Design review of the part built by this model. Coordinates are the model's own, in mm. Round coordinates to 2 decimals unless told otherwise and drop trailing zeros. Order: outer loops, then holes, each group sorted by start corner. A loop starts at its lowest first (then second) coordinate and runs counter-clockwise, first axis right, second up. Notation, with made-up numbers: M -24,57 L 22,57 A17 ccw 22,72 Z; hole C 69,-33 d10. An arc over 180 degrees is marked long. Use a Markdown table: item, result. Add a question column.
(1) Take a section at A-A (x = -104.5). Write out the cut boundary in (y, z).
(2) For pin 1 (3 mm diameter, centred on y = -21.5, z = 4, fed in from +X); pin 2 (3 mm diameter, centred on x = 296.5, z = 2, fed in from -Y), all flat-tipped, find the tip position at first contact; note any pin that passes through.
(3) To check wall thickness, follow probe 1 along X at (y, z) = (11, 3.75); probe 2 along Y at (x, z) = (196, 1.8); probe 3 along X at (y, z) = (-14.5, 4.55). State the ranges of each line that lie inside material, in increasing order. Write a range as from..to.
(4) Take a section at B-B (z = 3). Count the separate pieces of the cut face and the enclosed holes in it, then the cut area to 3 significant figures.
(5) Take a section at C-C (y = 32.5). Write out the cut boundary in (x, z).
Solid Edge part; units mm, degrees
sketch "Sketch1" plane through (0, 0, 0) normal (0, 0, 1) x (1, 0, 0)
  line L0 (-210, 6.5) -> (-190, 6.5)
  line L1 (-190, 6.5) -> (-190, 12.5)
  line L2 (-190, 12.5) -> (-210, 12.5)
  line L3 (-210, 12.5) -> (-210, 6.5)
  line L4 (-110, 6.5) -> (-90, 6.5)
  line L5 (-90, 6.5) -> (-90, 12.5)
  line L6 (-90, 12.5) -> (-110, 12.5)
  line L7 (-110, 12.5) -> (-110, 6.5)
  line L8 (-10, 6.5) -> (10, 6.5)
  line L9 (10, 6.5) -> (10, 12.5)
  line L10 (10, 12.5) -> (-10, 12.5)
  line L11 (-10, 12.5) -> (-10, 6.5)
  line L12 (90, 6.5) -> (110, 6.5)
  line L13 (110, 6.5) -> (110, 12.5)
  line L14 (110, 12.5) -> (90, 12.5)
  line L15 (90, 12.5) -> (90, 6.5)
  line L16 (190, 6.5) -> (210, 6.5)
  line L17 (210, 6.5) -> (210, 12.5)
  line L18 (210, 12.5) -> (190, 12.5)
  line L19 (190, 12.5) -> (190, 6.5)
  line L20 (-294, -37.5) -> (294, -37.5)
  line L21 (294, -12.5) -> (294, -37.5)
  line L22 (300, -12.5) -> (294, -12.5)
  line L23 (300, -12.5) -> (300, 12.5)
  line L24 (294, 12.5) -> (300, 12.5)
  line L25 (294, 37.5) -> (294, 12.5)
  line L26 (294, 37.5) -> (100, 37.5)
  line L27 (-100, 37.5) -> (100, 37.5)
  line L28 (-100, 37.5) -> (-294, 37.5)
  line L29 (-294, 12.5) -> (-294, 37.5)
  line L30 (-300, 12.5) -> (-294, 12.5)
  line L31 (-300, 12.5) -> (-300, -12.5)
  line L32 (-294, -12.5) -> (-300, -12.5)
  line L33 (-294, -37.5) -> (-294, -12.5)
  dimension "D1" = 210
  dimension "D2" = 190
  dimension "D3" = 110
  dimension "D4" = 90
  dimension "D5" = 90
  dimension "D6" = 110
  dimension "D7" = 190
  dimension "D8" = 210
  dimension "D9" = 190
  dimension "D10" = 90
  dimension "D11" = 110
  dimension "D12" = 210
extrude "Protrusion1" add sketch "Sketch1" along normal blind 6
Verdict:
| question | item | result |
|---|---|---|
| 1 | outline | M -37.5,0 L 6.5,0 L 6.5,6 L -37.5,6 Z; M 12.5,0 L 37.5,0 L 37.5,6 L 12.5,6 Z |
| 2 | pin 1 | stops at x = 294 |
| 2 | pin 2 | stops at y = -12.5 |
| 3 | probe 1 | x = -300..-210, -190..-110, -90..-10, 10..90, 110..190, 210..300 |
| 3 | probe 2 | y = -37.5..6.5, 12.5..37.5 |
| 3 | probe 3 | x = -294..294 |
| 4 | separate pieces | 1 |
| 4 | enclosed holes | 5 |
| 4 | area | 43,800 mm^2 |
| 5 | outline | M -294,0 L 294,0 L 294,6 L -294,6 Z |
